Check sheet for the drawn part. Datum: minimum x, y, z corner. Units: mm. A direction names the side the tool comes from. Coordinates: 2 decimals unless noted, no trailing zeros. Write each loop counter-clockwise with the first axis right and the second up, starting at its lowest first coordinate (ties: lowest second). Pieces come first, ordered by that corner, then holes. Notation, with made-up numbers: (-17, -39) -> (26, -39) arc R30 cw to (26, -3) -> close; hole circle Ø4 at (-7, 72). An arc over 180 degrees is marked (long way). Answer in a Markdown table with one row per item. Add a question column.
Q1. Section check D-D, the plane z = 12.5. Record the boundary of the cut face in (x, y) (3 decimals), and give its area (3 significant figures).
Q2. Thickness scan on line 1 (Z direction, x = 15, y = 25.5); line 2 (X direction, y = 22, z = 12.5); line 3 (Y direction, x = 12.5, z = 12.5). Record the ranges inside material, lowest first.
Q3. Section check C-C, the plane y = 23. Record the boundary of the cut face in (x, z).
Q4. Section check A-A, the plane y = 15. Record the boundary of the cut face in (x, z) (3 decimals), and give its area (3 significant figures).
Q5. Gauge pin test, flat ends, axial feed: P1, Ø8, axis at x = 9.5, z = 16.5, coming from the -Y side; P2, Ø1.5, axis at y = 20, z = 9, coming from the +X side; P3, Ø10, axis at x = 16.5, z = 4, coming from the -Y side; P4, Ø4, axis at y = 13.5, z = 17, coming from the -X side (3 decimals). Record the tip position at first contact, or that the pin passes through.
Q6. Tool access check on the marked faces 1 and 2. Record the directions out of +Z, -Z, +X, -X, +Y, -Y that give a thin tool (end or side, any length) a straight path to the whole face; none if there is none.
Q7. Release check for a two-part mould opening along Z. For the marked faces 3, 4, 5 and 6 record: pulls with the +Z half, pulls with the -Z half, needs draft (parallel to the pull), parting line crosses it, or undercut.
Q8. Section check B-B, the plane x = 15. Record the boundary of the cut face in (y, z) (3 decimals), and give its area (3 significant figures).
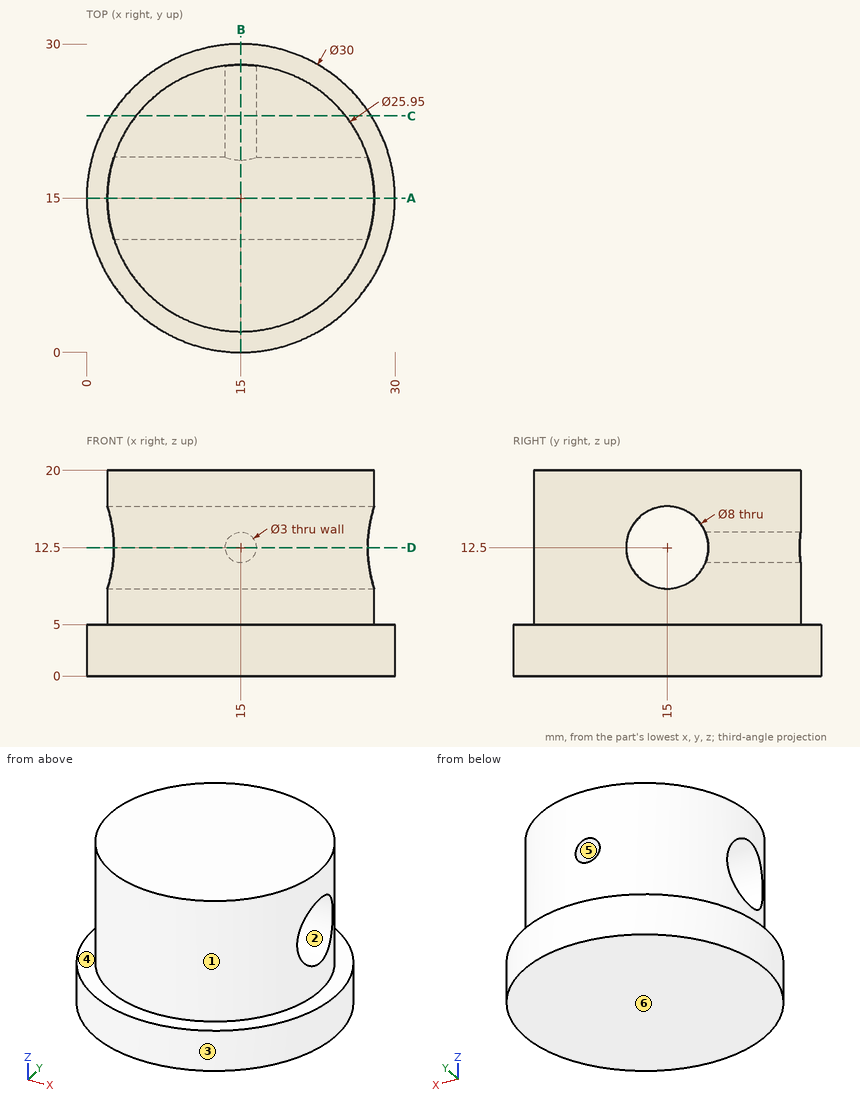
Calculated:
| question | item | result |
|---|---|---|
| 1 | outline | (2.657, 11) arc R12.975 ccw to (27.343, 11) -> close; (2.657, 19) -> (13.5, 19) -> (13.5, 27.888) arc R12.975 ccw to start; (16.5, 19) -> (27.343, 19) arc R12.975 ccw to (16.5, 27.888) -> close |
| 1 | area | 298 mm² |
| 2 | line 1 | z = 0 to 11, 14 to 20 |
| 2 | line 2 | x = 4.08 to 13.5, 16.5 to 25.92 |
| 2 | line 3 | y = 2.27 to 11, 19 to 27.73 |
| 3 | outline | (2.31, 0) -> (27.69, 0) -> (27.69, 5) -> (25.22, 5) -> (25.22, 20) -> (4.78, 20) -> (4.78, 5) -> (2.31, 5) -> close; hole circle Ø3 at (15, 12.5) |
| 4 | outline | (0, 0) -> (30, 0) -> (30, 5) -> (27.975, 5) -> (27.975, 8.5) -> (2.025, 8.5) -> (2.025, 5) -> (0, 5) -> close; (2.025, 16.5) -> (27.975, 16.5) -> (27.975, 20) -> (2.025, 20) -> close |
| 4 | area | 332 mm² |
| 5 | P1 | stops at y = 2.11 |
| 5 | P2 | stops at x = 27.26 |
| 5 | P3 | stops at y = 0 |
| 5 | P4 | stops at x = 2.025 |
| 6 | face 1 | +Z |
| 6 | face 2 | +X, -X |
| 7 | face 3 | needs draft |
| 7 | face 4 | pulls with the +Z half |
| 7 | face 5 | undercut |
| 7 | face 6 | pulls with the -Z half |
| 8 | outline | (0, 0) -> (30, 0) -> (30, 5) -> (27.975, 5) -> (27.975, 11) -> (18.708, 11) arc R4 cw (long way) to (18.708, 14) -> (27.975, 14) -> (27.975, 20) -> (2.025, 20) -> (2.025, 5) -> (0, 5) -> close |
| 8 | area | 462 mm² |
